The listing builds one solid part. Answer for the finished solid, in the listing's coordinates (mm). A direction names the side the tool comes from. Round coordinates to 2 decimals unless told otherwise and drop trailing zeros. Write each loop counter-clockwise with the first axis right and the second up, starting at its lowest first coordinate (ties: lowest second). Pieces come first, ordered by that corner, then holes. Notation, with made-up numbers: (44, 15.25) - (62, 15.25) arc R22 ccw to (62, 27.25) - close; hole circle Ø6 at (55.5, -22.5). An arc over 180 degrees is marked (long way). Use a Markdown table: item, result. Add a question column.
1) A tool of negligible diameter and unlimited length cuts with its end or side. For faces 4 (the flat face through (17.74, 575.52, -4.93)), 5 (the flat face through (12.23, 562.213, -3.594)), from which of +Z, -Z, +X, -X, +Y, -Y can it reach the whole face along a straight path? Write none if from no direction.
2) Find the intervals of material crossed by probe 1 along Z at (x, y) = (-8, 571.5); probe 2 along Z at (x, y) = (10, 592.5); probe 3 along Z at (x, y) = (19, 592), in increasing order. Write a range as from..to.
3) A cutting plane is placed at C-C (x = -16). Give the vertices of the cut face in (y, z).
4) A cutting plane is placed at B-B (z = 5.75). Give the vertices of the cut face in (x, y) (3 decimals), then the cut area to 3 significant figures.
5) A cutting plane is placed at A-A (y = 590.5). Give the vertices of the cut face in (x, z), then the cut area to 3 significant figures.
6) Determine the mould class of faces 1 (the flat face through (-17.26, 575.52, -5.07)), 2 (the cylindrical face through (-1.71, 597.3, 0.38)), 3 (the flat face through (9.925, 636.763, 3.819)) for opening direction X: +X half, -X half, draft (parallel to the pull), parting line (faces both ways), or undercut.
7) A cutting plane is placed at D-D (y = 659). Give the vertices of the cut face in (x, z) (1 decimal).
8) Each of these flat-tipped pins is pushed along its axis until it touches: P1, Ø1, axis at x = -0.5, z = 0.5, coming from the -Y side; P2, Ø6, axis at x = 19.5, y = 622.5, coming from the +Z side; P3, Ø6, axis at x = -9.5, y = 593, coming from the -Z side; P4, Ø10, axis at x = -25.5, z = 5.5, coming from the -Y side. Where does it stop, or does it pass through?
```python
from build123d import *

# Parameters (mm, degrees)
SWEEP_1_DEPTH            = 610
CUT_EXTRUDE_2_DEPTH      = 12
SKETCH_21_R              = 1.75
CUT_EXTRUDE_3_DEPTH      = 600
CUT_EXTRUDE_4_DEPTH      = 691.959477934
CUT_EXTRUDE_4_DEPTH_BACK = 691.959477934
SKETCH_26_W              = 70
SKETCH_26_H              = 530
CUT_EXTRUDE_5_DEPTH      = 41


# Read off the part's stored shape, not the designer's step: 扫描1
with BuildPart() as part:
    # 扫描1 outline → 扫描1 (new body)
    with BuildSketch(Plane(origin=(0, 0, 0), x_dir=(1, 0, 0), z_dir=(0, 1, 0))):
        Polygon((-35, 0), (35, 0), (0, 10), align=None)
    sweep_1 = extrude(amount=SWEEP_1_DEPTH)

    # 草图1 → 放样1 section 0
    with BuildSketch(Plane.XY, mode=Mode.PRIVATE) as loft_1_s0:
        with BuildLine():
            Line((-35, 610), (0, 690))
            Line((0, 690), (35, 610))
            Line((35, 610), (-35, 610))
        make_face()
    loft_1 = loft([Vertex(0, 610, -10), loft_1_s0.sketch])

    # 镜向1: 扫描1, 放样1 across plane
    add(sweep_1.mirror(Plane.XY))
    add(loft_1.mirror(Plane.XY))

    # 草图19 → 切除-拉伸2 (cut)
    with BuildSketch(Plane.XZ):
        Polygon((0, -10), (35, 0), (0, 10), (-35, 0), align=None)
    extrude(amount=-CUT_EXTRUDE_2_DEPTH, mode=Mode.SUBTRACT)

    # 草图21 → 切除-拉伸3 (cut)
    with BuildSketch(Plane.XZ.offset(-12)):
        with Locations(Location((0, 0, 0), (0, 0, 270))):
            Circle(SKETCH_21_R)
    extrude(amount=-CUT_EXTRUDE_3_DEPTH, mode=Mode.SUBTRACT)

    # 草图26 → 切除-拉伸4 (cut, two sides: drawn at the far end of the back side and taken through both)
    with BuildSketch(Plane.XY.offset(-CUT_EXTRUDE_4_DEPTH_BACK)):
        with Locations((0, 277)):
            Rectangle(SKETCH_26_W, SKETCH_26_H)
    extrude(amount=CUT_EXTRUDE_4_DEPTH + CUT_EXTRUDE_4_DEPTH_BACK, mode=Mode.SUBTRACT)

    # 草图27 → 切除-拉伸5 (cut)
    with BuildSketch(Plane.XZ.offset(-542)):
        Polygon((0, -7.087956044), (24.807846155, 0), (0, 7.087956044), (-24.807846155, 0), align=None)
    extrude(amount=-CUT_EXTRUDE_5_DEPTH, mode=Mode.SUBTRACT)


solid = part.part
```
Entries:
| question | item | result |
|---|---|---|
| 1 | face 4 | -Z, +X, +Y, -Y |
| 1 | face 5 | -Y |
| 2 | probe 1 | z = -7.71..-4.8, 4.8..7.71 |
| 2 | probe 2 | z = -7.14..7.14 |
| 2 | probe 3 | z = -4.57..4.57 |
| 3 | outline | (542, -5.43) - (610, -5.43) - (653.43, 0) - (610, 5.43) - (542, 5.43) - (542, 2.52) - (583, 2.52) - (583, -2.52) - (542, -2.52) - close |
| 4 | outline | (-14.875, 542) - (-4.683, 542) - (-4.683, 583) - (4.683, 583) - (4.683, 542) - (14.875, 542) - (14.875, 610) - (0, 644) - (-14.875, 610) - close |
| 4 | area | 2,140 mm² |
| 5 | outline | (-35, 0) - (0, -10) - (35, 0) - (0, 10) - close; hole circle Ø3.5 at (0, 0) |
| 5 | area | 690 mm² |
| 6 | face 1 | -X half |
| 6 | face 2 | undercut |
| 6 | face 3 | +X half |
| 7 | outline | (-13.6, 0) - (0, -3.9) - (13.6, 0) - (0, 3.9) - close |
| 8 | P1 | stops at y = 612 |
| 8 | P2 | stops at z = 3.8 |
| 8 | P3 | stops at z = -8.14 |
| 8 | P4 | stops at y = 542 |
